Geometry check sheet. Reference: drawing and pictorial views, mm from the part's lowest x, y, z. Coordinates: 2 decimals unless noted, no trailing zeros. Loops run counter-clockwise (first coordinate to the right, second up) from the corner with the lowest first, then second, coordinate; pieces in that order, holes last. Notation, with made-up numbers: (17.25, 38) -> (53.25, 38) arc R14 cw to (53.25, 43) -> close; hole circle Ø5 at (41.25, -26.75). An arc over 180 degrees is marked (long way). Use CSV: the item, a comma, the result in double quotes.
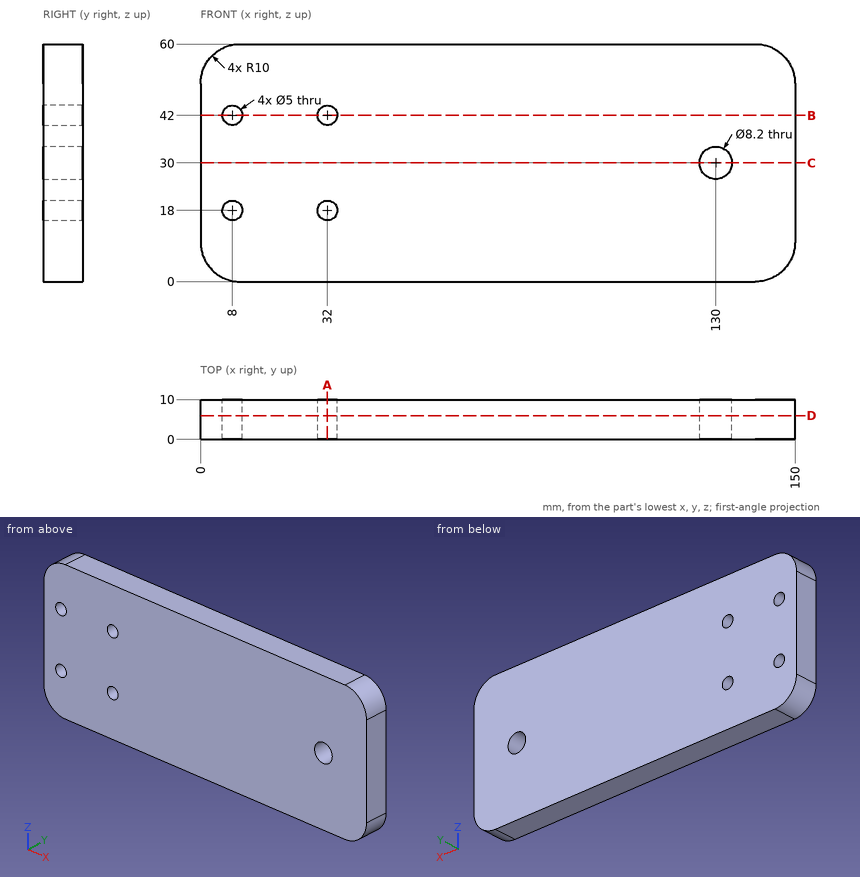
1) Cross-section at A-A on x = 32. Record the boundary of the cut face in (y, z).
Answer below:
outline,"(0, 0) -> (10, 0) -> (10, 15.5) -> (0, 15.5) -> close; (0, 20.5) -> (10, 20.5) -> (10, 39.5) -> (0, 39.5) -> close; (0, 44.5) -> (10, 44.5) -> (10, 60) -> (0, 60) -> close"
2) Cross-section at B-B on z = 42. Record the boundary of the cut face in (x, y), and give its area (3 significant figures).
Answer below:
outline,"(0, 0) -> (5.5, 0) -> (5.5, 10) -> (0, 10) -> close; (10.5, 0) -> (29.5, 0) -> (29.5, 10) -> (10.5, 10) -> close; (34.5, 0) -> (150, 0) -> (150, 10) -> (34.5, 10) -> close"
area,"1,400 mm²"
3) Cross-section at D-D on y = 6. Record the boundary of the cut face in (x, z), and give its area (3 significant figures).
Answer below:
outline,"(0, 10) arc R10 ccw to (10, 0) -> (140, 0) arc R10 ccw to (150, 10) -> (150, 50) arc R10 ccw to (140, 60) -> (10, 60) arc R10 ccw to (0, 50) -> close; hole circle Ø5 at (8, 18); hole circle Ø5 at (8, 42); hole circle Ø5 at (32, 18); hole circle Ø5 at (32, 42); hole circle Ø8.2 at (130, 30)"
area,"8,780 mm²"
4) Thickness scan on line 1 along Z through (x, y) = (130, 4); line 2 along X through (y, z) = (5.75, 3.5); line 3 along X through (y, z) = (7, 5.5). Record the ranges inside material, lowest first. Write a range as from..to.
Answer below:
line 1,"z = 0..25.9, 34.1..60"
line 2,"x = 2.4..147.6"
line 3,"x = 1.07..148.93"
5) Cross-section at C-C on z = 30. Record the boundary of the cut face in (x, y), and give its area (3 significant figures).
Answer below:
outline,"(0, 0) -> (125.9, 0) -> (125.9, 10) -> (0, 10) -> close; (134.1, 0) -> (150, 0) -> (150, 10) -> (134.1, 10) -> close"
area,"1,420 mm²"
